For this review, take the finished solid that the model builds, in its own axes (mm). Face numbers are marked on the shaded views. A direction names the side the tool comes from. Coordinates: 2 decimals unless noted, no trailing zeros. Loops run counter-clockwise (first coordinate to the right, second up) from the corner with the lowest first, then second, coordinate; pieces in that order, holes last. Notation, with made-up numbers: M -33,31.25 L -23,31.25 A22 cw -23,56.25 Z; hole C -37,7.5 d2. An arc over 180 degrees is marked long. Write item = value, one per line.
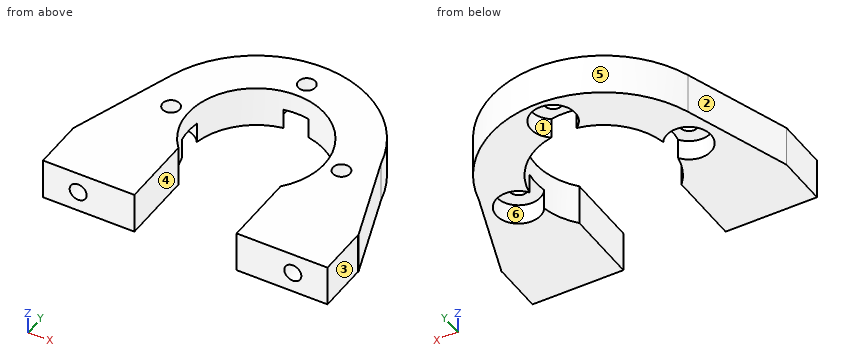
Autodesk Inventor part; units mm, degrees
ref_plane "YZ Plane" through (0, 0, 0) normal (1, 0, 0) x (0, 1, 0)
ref_plane "XZ Plane" through (0, 0, 0) normal (0, 1, 0) x (-1, 0, 0)
ref_plane "XY Plane" through (0, 0, 0) normal (0, 0, 1) x (1, 0, 0)
sketch "Sketch1" plane through (0, 0, 0) normal (0, 0, 1) x (1, 0, 0)
  circle A0 centre (0, 0) radius 10
  arc A1 (13.1244, -10) -> (-13.1244, -10) centre (0, 0) ccw
  line L0 (13.1244, -10) -> (25, -10)
  line L1 (25, -10) -> (0, -10)
  line L2 (-13.1244, -10) -> (-25, -10)
  line L3 (0, 0) -> (0, -17.5)
  line L4 (0, -17.5) -> (-25, -17.5)
  line L5 (-25, -17.5) -> (-25, -10)
  line L6 (25, -10) -> (25, -17.5)
  line L7 (25, -17.5) -> (0, -17.5)
  line L8 (0, 0) -> (-12.5, 0)
  circle A2 centre (-12.5, 0) radius 1.25
  line L9 (0, 0) -> (0, 12.5)
  circle A3 centre (0, 12.5) radius 1.25
  circle A4 centre (12.5, 0) radius 1.25
  circle A5 centre (0, -12.5) radius 1.25
  circle A6 centre (12.5, 0) radius 3.25
  circle A7 centre (-12.5, 0) radius 3.25
  line L10 (0, 0) -> (2.11, 2.11)
  line L11 (0, 0) -> (2.984, 0) construction
  circle A8 centre (0, 12.5) radius 3.25
  circle A9 centre (0, -12.5) radius 3.25
  dimension "d0" = 20
  dimension "d1" = 33
  dimension "d2" = 25
  dimension "d3" = 25
  dimension "d4" = 17.5
  dimension "d5" = 25
  dimension "d6" = 12.5
  dimension "d7" = 2.5
  dimension "d8" = 12.5
  dimension "d9" = 2.5
  dimension "d15" = 6.5
  dimension "d16" = 45
  dimension "d17" = 6.5
  dimension "d18" = 6.5
extrude "Extrusion1" add sketch "Sketch1" along normal blind 6 contours A0 A6 | A0 A8 A7 A9 L3 L4 L5 L2 A1 L1 A6 | A0 A8 | A9 L1 A0 | L3 A5 A9 A0 | L1 A9 L3 A5 | L1 L0 L6 L7 L3 A9 | A5 L3 | L3 A5 | A0 A7 picked at (10.6028, 1.4923)
fillet "Fillet1" radius 5 2 edges at (13.1244, -10, 3) (-13.1244, -10, 3)
sketch "Sketch2" plane through (0, 0, 0) normal (0, 0, -1) x (-1, 0, 0)
  circle A0 centre (0, 12.5) radius 1.25
  line L0 (0, 0) -> (-3.0567, 0)
  circle A1 centre (0, -12.5) radius 1.25
extrude "Extrusion2" cut sketch "Sketch2" against normal blind 10 contours A1
sketch "Sketch3" plane through (0, 0, 0) normal (0, 0, -1) x (-1, 0, 0)
  circle A0 centre (-12.5, 0) radius 1.25
  circle A1 centre (0, -12.5) radius 1.25
  circle A2 centre (0, 0) radius 10
  circle A3 centre (-12.5, 0) radius 1.25
  circle A4 centre (0, 12.5) radius 1.25
  circle A5 centre (12.5, 0) radius 1.25
  line L0 (25, -17.5) -> (-25, -17.5)
  line L1 (25, -10) -> (25, -17.5)
  line L2 (20.9105, -10) -> (25, -10)
  arc A6 (16.0476, -3.8372) -> (20.9105, -10) centre (20.9105, -5) ccw
  arc A7 (16.0476, -3.8372) -> (-16.0476, -3.8372) centre (0, 0) ccw
  arc A8 (-20.9105, -10) -> (-16.0476, -3.8372) centre (-20.9105, -5) ccw
  line L3 (-25, -10) -> (-20.9105, -10)
  line L4 (-25, -17.5) -> (-25, -10)
  circle A9 centre (-12.5, 0) radius 3.25
  circle A10 centre (0, 12.5) radius 3.25
  circle A11 centre (12.5, 0) radius 1.25
  circle A12 centre (12.5, 0) radius 3.25
  circle A13 centre (0, -12.5) radius 3.25
  dimension "d19" = 6.5
  dimension "d20" = 6.5
  dimension "d21" = 6.5
  dimension "d22" = 6.5
extrude "Extrusion3" cut sketch "Sketch3" against normal blind 3 contours A2 A12 | A2 A12 | A10 A2 | A2 A10 | A13 A2 | A2 A13 | A9 A2 | A2 A9
sketch "Sketch4" plane through (0, 0, 0) normal (0, 0, -1) x (-1, 0, 0)
  arc A0 (16.0476, -3.8372) -> (-16.0476, -3.8372) centre (0, 0) ccw
  line L0 (-25, -10) -> (-20.9105, -10)
  line L1 (-16.0476, 3.8372) -> (-20.9105, -10)
  line L2 (15.5959, 5.3868) -> (20.9105, -10)
  arc A1 (16.0476, -3.8372) -> (20.9105, -10) centre (20.9105, -5) ccw
  arc A2 (-20.9105, -10) -> (-16.0476, -3.8372) centre (-20.9105, -5) ccw
extrude "Extrusion4" add sketch "Sketch4" against normal up to surface (6 mm away)
sketch "Sketch5" plane through (-25, -17.5, 0) normal (0, -1, 0) x (1, 0, 0)
  line L0 (0, 6) -> (50, 6)
  line L1 (0, 0) -> (50, 0)
  circle A0 centre (40.75, 3) radius 1.25
  circle A1 centre (9.25, 3) radius 1.25
  point P0 (25, 0)
  dimension "d27" = 2.5
extrude "Extrusion5" cut sketch "Sketch5" against normal blind 14
sketch "Sketch6" plane through (-25, -17.5, 0) normal (0, -1, 0) x (1, 0, 0)
  circle A0 centre (9.25, 3) radius 1.25
  circle A1 centre (40.75, 3) radius 1.25
  point P0 (25, 0)
  dimension "d30" = 31.5
sketch "Sketch7" plane through (-25, -17.5, 0) normal (0, -1, 0) x (1, 0, 0)
  line L0 (32.5, -8.9217) -> (17.5, -8.9217)
  line L1 (17.5, -8.9217) -> (17.5, 8.9217)
  line L2 (17.5, 8.9217) -> (32.5, 8.9217)
  line L3 (32.5, 8.9217) -> (32.5, -8.9217)
  line L4 (32.5, -8.9217) -> (17.5, 8.9217) construction
  line L5 (17.5, -8.9217) -> (32.5, 8.9217) construction
  point P0 (25, 0)
  dimension "d31" = 15
extrude "Extrusion6" cut sketch "Sketch7" against normal blind 14
sketch "Sketch8" plane through (-25, -10, 6) normal (0, 1, 0) x (1, 0, 0)
  line L0 (9.4041, 6) -> (41.0476, 6)
  line L1 (4.0895, 6) -> (4.0895, 0)
  line L2 (9.4041, 6) -> (4.0895, 6)
  line L3 (4.0895, 6) -> (4.0895, 0)
  line L4 (4.0895, 0) -> (9.4041, 0)
  line L5 (9.4041, 0) -> (9.4041, 6)
  line L6 (45.8371, 0) -> (50, 0)
  line L7 (50, 0) -> (50, 6)
  line L8 (50, 6) -> (45.8371, 6)
  line L9 (45.8371, 6) -> (45.8371, 0)
  line L10 (0, 0) -> (4.0895, 0)
  line L11 (4.0895, 0) -> (4.0895, 6)
  line L12 (4.0895, 6) -> (0, 6)
  line L13 (0, 6) -> (0, 0)
  point P0 (25, 6)
extrude "Extrusion7" cut sketch "Sketch8" against normal blind 14 contours L1 L10 L13 L12 | L9 L8 L7 L6
properties part number "ROTATION2"
Q1. Add section D-D (y = 13). Write out the cut boundary in (x, z), and give its area (3 significant figures).
Solved:
outline = M -10.16,0 L -3.21,0 L -3.21,3 L -1.15,3 L -1.15,6 L -10.16,6 Z; M 1.15,3 L 3.21,3 L 3.21,0 L 10.16,0 L 10.16,6 L 1.15,6 Z
area = 95.8 mm²
Q2. Add section C-C (y = -7.5). Write out the cut boundary in (x, z), and give its area (3 significant figures).
Solved:
outline = M -20.05,0 L -7.5,0 L -7.5,6 L -20.05,6 Z; M 7.5,0 L 20.03,0 L 20.03,6 L 7.5,6 Z; hole C -15.75,3 d2.5; hole C 15.75,3 d2.5
area = 141 mm²
Q3. For pin 1 Ø1.5 at (y, z) = (6, 1) entering from +X; pin 2 Ø1.8 at (y, z) = (-15, 1.5) entering from +X; pin 3 Ø6 at (x, y) = (-12.5, 0) entering from -Z, all flat-tipped, find the tip position at first contact; note any pin that passes through.
Solved:
pin_1 = 15.64
pin_2 = 20.84
pin_3 = 3
Q4. For line 1 along X through (y, z) = (-3, 2.35); line 2 along X through (y, z) = (-4, 3.65); line 3 along X through (y, z) = (12.5, 4.6), list the stretches that pass through material, from the lowest coordinate up.
Solved:
line_1 = -18.49 to -13.75, -11.25 to -9.54, 9.54 to 11.25, 13.75 to 18.45
line_2 = -18.84 to -16.82, -14.68 to -9.17, 9.17 to 14.68, 16.82 to 18.8
line_3 = -10.77 to -1.25, 1.25 to 10.77
Q5. Add section A-A (x = 0). Write out the cut boundary in (y, z).
Solved:
outline = M 10,3 L 11.25,3 L 11.25,6 L 10,6 Z; M 13.75,3 L 15.75,3 L 15.75,0 L 16.5,0 L 16.5,6 L 13.75,6 Z
Q6. Add section B-B (z = 5.35). Write out the cut boundary in (x, y).
Solved:
outline = M -20.91,-17.5 L -7.5,-17.5 L -7.5,-6.61 A10 cw long 7.5,-6.61 L 7.5,-17.5 L 20.84,-17.5 L 20.84,-10 L 20.91,-10 L 16.05,3.84 A16.5 ccw -15.6,5.39 L -20.91,-10 Z; hole C -12.5,0 d2.5; hole C 0,12.5 d2.5; hole C 12.5,0 d2.5
Q7. Draft analysis for pull direction X (two halves, no side actions). For the marked faces 1, 2 and 3, state which applies: +X half, -X half, draft (parallel to the pull), parting line (faces both ways), or undercut.
Solved:
face_1 = undercut
face_2 = -X half
face_3 = +X half
Q8. Machinability: for the marked faces 4, 5 and 6, which of the approach directions +Z, -Z, +X, -X, +Y, -Y give a long, thin tool a straight path to every point of the face, cutting with its end or side? Answer none if there is none.
Solved:
face_4 = +Z, -Z, -Y
face_5 = +Z, -Z, +Y
face_6 = -Z
